Part print with two shaded views. Sizes in mm from the minimum x, y, z corner. A direction names the side the tool comes from. Give positions to 0.01 mm unless a question says otherwise; leave off trailing zeros. Write each loop counter-clockwise with the first axis right and the second up, starting at its lowest first coordinate (ties: lowest second). Pieces come first, ordered by that corner, then holes. Notation, with made-up numbers: (33, -18) -> (79, -18) arc R11 ccw to (79, 0) -> close; hole circle Ø2 at (88.5, 63). An arc over 180 degrees is marked (long way). Answer in a Markdown table with one row per item. Add a question column.
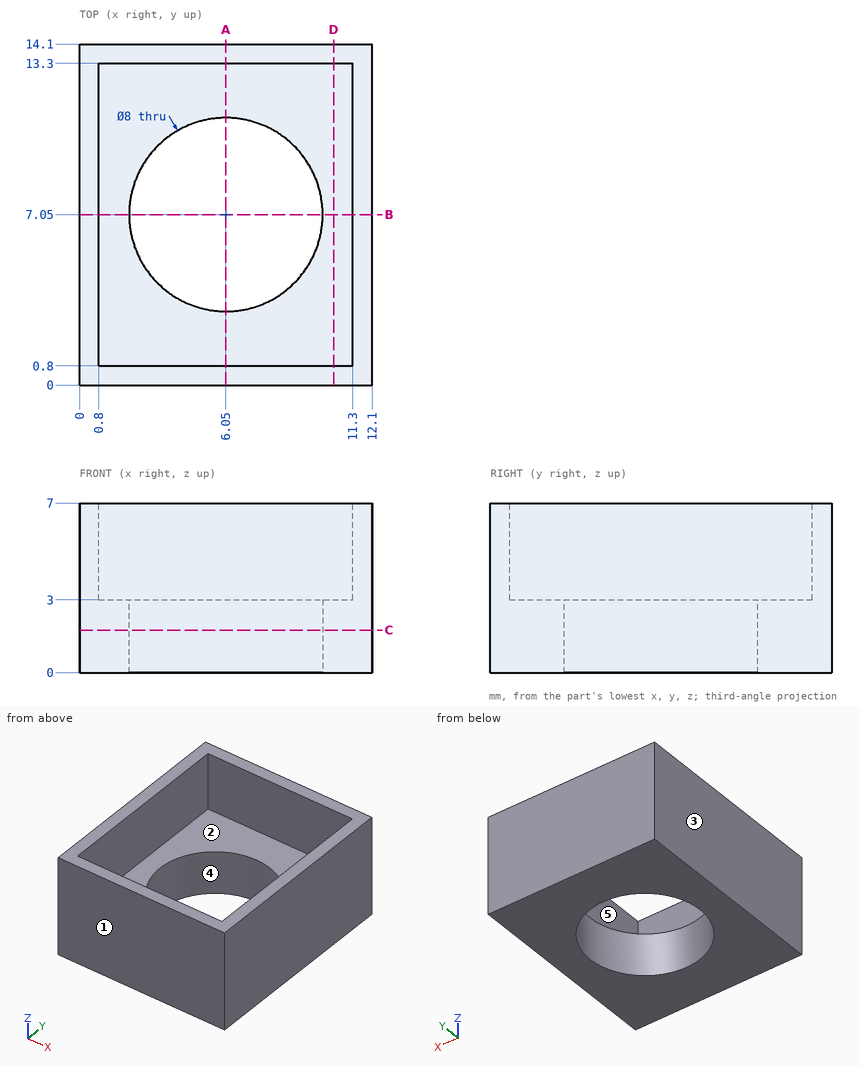
Item 1: Which spindle directions (+Z, -Z, +X, -X, +Y, -Y) get a long thin tool onto all of the face, cutting with end or side? Do the marked faces 4 and 5. Say none if no direction does.
Item 2: Slice it at C-C, the plane z = 1.75. List the corners of the cut face in (x, y), then the cut area to 3 significant figures.
Item 3: Probe L1, parallel to Y at x = 6.05, z = 1.85; L2, parallel to Y at x = 9.75, z = 5.25; L3, parallel to X at y = 10, z = 4.75. List the from-to ranges inside material, lowest first. Write a range as from..to.
Item 4: Slice it at A-A, the plane x = 6.05. List the corners of the cut face in (y, z).
Item 5: Drop flat-ended pins along their axis: pin 1 Ø3 at (y, z) = (8.5, 6) entering from -X; pin 2 Ø2 at (x, y) = (5, 10) entering from +Z; pin 3 Ø3 at (x, y) = (5.5, 6.5) entering from +Z. Give the stop position or say it passes through.
Item 6: Slice it at D-D, the plane x = 10.5. List the corners of the cut face in (y, z).
Item 7: Slice it at B-B, the plane y = 7.05. List the corners of the cut face in (x, z), then the cut area to 3 significant figures.
Item 8: Mould opens along X. For the marked faces 1, 2 and 3 say: released by +X, released by -X, zero draft, split by the parting line, or undercut.
Answer key:
| question | item | result |
|---|---|---|
| 1 | face 4 | +Z, -Z |
| 1 | face 5 | +Z |
| 2 | outline | (0, 0) -> (12.1, 0) -> (12.1, 14.1) -> (0, 14.1) -> close; hole circle Ø8 at (6.05, 7.05) |
| 2 | area | 120 mm² |
| 3 | L1 | y = 0..3.05, 11.05..14.1 |
| 3 | L2 | y = 0..0.8, 13.3..14.1 |
| 3 | L3 | x = 0..0.8, 11.3..12.1 |
| 4 | outline | (0, 0) -> (3.05, 0) -> (3.05, 3) -> (0.8, 3) -> (0.8, 7) -> (0, 7) -> close; (11.05, 0) -> (14.1, 0) -> (14.1, 7) -> (13.3, 7) -> (13.3, 3) -> (11.05, 3) -> close |
| 5 | pin 1 | stops at x = 0 |
| 5 | pin 2 | stops at z = 3 |
| 5 | pin 3 | passes through |
| 6 | outline | (0, 0) -> (14.1, 0) -> (14.1, 7) -> (13.3, 7) -> (13.3, 3) -> (0.8, 3) -> (0.8, 7) -> (0, 7) -> close |
| 7 | outline | (0, 0) -> (2.05, 0) -> (2.05, 3) -> (0.8, 3) -> (0.8, 7) -> (0, 7) -> close; (10.05, 0) -> (12.1, 0) -> (12.1, 7) -> (11.3, 7) -> (11.3, 3) -> (10.05, 3) -> close |
| 7 | area | 18.7 mm² |
| 8 | face 1 | zero draft |
| 8 | face 2 | undercut |
| 8 | face 3 | released by -X |
